Read the model definition and answer for the solid it produces. Units are mm, in the model's axes. A direction names the side the tool comes from. Give positions to 0.01 mm unless a question says otherwise; leave off trailing zeros. Loops run counter-clockwise (first coordinate to the right, second up) from the corner with the lowest first, then second, coordinate; pieces in that order, holes last. Notation, with made-up numbers: (36, 6.25) -> (79, 6.25) arc R23 cw to (79, 14.25) -> close; hole circle Ø9 at (42.25, 68.5). An arc over 180 degrees is marked (long way). Answer as CSV lines item,"result". Start each with the question number.
Autodesk Inventor part; units mm, degrees
ref_plane "YZ Plane" through (0, 0, 0) normal (1, 0, 0) x (0, 1, 0)
ref_plane "XZ Plane" through (0, 0, 0) normal (0, 1, 0) x (-1, 0, 0)
ref_plane "XY Plane" through (0, 0, 0) normal (0, 0, 1) x (1, 0, 0)
sketch "Sketch1" plane through (0, 0, 0) normal (0, 1, 0) x (-1, 0, 0)
  line L0 (0, 0) -> (60, 0)
  line L1 (60, 0) -> (60, -100)
  line L2 (60, -100) -> (0, -100)
  line L3 (0, -100) -> (0, 0)
  dimension "d0" = 100
  dimension "d1" = 60
extrude "Extrusion1" add sketch "Sketch1" along normal blind 40
sketch "Sketch2" plane through (0, 0, 0) normal (1, 0, 0) x (0, 0, -1)
  line L0 (0, 0) -> (37.6485, 44.8677)
  line L1 (0, 0) -> (58.5706, 0) construction
  line L2 (100, 40) -> (0, 40)
  line L3 (0, 40) -> (0, 0)
  point P0 (33.564, 40)
  dimension "d4" = 50
extrude "Extrusion2" cut sketch "Sketch2" against normal blind 70
sketch "Sketch3" plane through (0, 0, -100) normal (1, 0, 0) x (0, 0, -1)
  line L0 (0, 0) -> (-17, 0)
  line L1 (-100, 0) -> (0, 0)
  line L2 (0, 40) -> (-66.436, 40)
  line L3 (-17, 40) -> (-37, 40)
  line L4 (-37, 40) -> (-37, 10)
  line L5 (-37, 10) -> (-17, 10)
  line L6 (-17, 10) -> (-17, 40)
  dimension "d7" = 17
  dimension "d8" = 20
  dimension "d9" = 30
extrude "Extrusion3" add sketch "Sketch3" along normal blind 20
sketch "Sketch4" plane through (0, 10, -63) normal (0, 0, 1) x (1, 0, 0)
  line L0 (0, 30) -> (-60, 30)
  line L1 (0, 30) -> (29.4147, 5.3181)
  line L2 (0, 30) -> (38.3982, 30) construction
  line L3 (0, 30) -> (20, 30)
  line L4 (0, 30) -> (20, 30)
  line L5 (20, 30) -> (20, 13.218)
  line L6 (20, 0) -> (20, 30)
  point P0 (0, -10)
  dimension "d12" = 40
extrude "Extrusion4" cut sketch "Sketch4" against normal blind 61.75
ref_plane "Work Plane1" through (-30, 0, -100) normal (1, 0, 0) x (0, 0, -1)
mirror "Mirror1" about plane through (-30, 0, -100) normal (1, 0, 0) of "Extrusion3", "Extrusion4"
sketch "Sketch5" plane through (0, 40, -63) normal (0.6428, 0.766, 0) x (0.766, -0.6428, 0)
  circle A0 centre (12.5, 10) radius 5
  point P0 (25.7115, -63)
  dimension "d16" = 10
extrude "Extrusion5" cut sketch "Sketch5" against normal blind 27
mirror "Mirror2" about plane through (-30, 0, -100) normal (1, 0, 0) of "Extrusion5"
sketch "Sketch6" plane through (20, 10, -83) normal (0, 0, -1) x (-1, 0, 0)
  line L0 (20, 30) -> (20, 0)
  line L1 (20, 30) -> (20, 20)
  line L2 (20, 20) -> (18.6004, 20)
  line L3 (18.6004, 20) -> (18.6004, 28.8256)
  line L4 (0, 13.218) -> (20, 30)
  point P0 (20, -10)
  point P1 (20, 20)
  dimension "d19" = 10
extrude "Extrusion6" cut sketch "Sketch6" against normal blind 38.25
mirror "Mirror3" about plane through (-30, 0, -100) normal (1, 0, 0) of "Extrusion6"
properties part number "taslak"
(1) Find section B-B on y = 32. Give the number of separate pieces and of enclosed holes in the cut face, then the cut area to 3 significant figures.
(2) Find section A-A on x = -22.5. Write down the section's boundary in (y, z).
(3) Find section C-C on z = -48. Write down the section's boundary in (x, y).
(4) The mould has two halves that part along X. Classify faces 4 (the face through (-70, 21, -83)), 5 (the face through (-72.897, 29.178, -68.416)), 6 (the face through (1.4, 34, -73)): pulls with the +X half, pulls with the -X half, needs draft (parallel to the pull), parting line crosses it, or undercut.
(5) A tool of negligible diameter and unlimited length cuts with its end or side. For faces 1 (the face through (10, 10, -73)), 2 (the face through (-61.4, 34, -73)), 3 (the face through (10, 21, -83)), from which of +Z, -Z, +X, -X, +Y, -Y can it reach the whole face along a straight path? Write none if from no direction.
(6) Find the intervals of material crossed by line 1 along X through (y, z) = (13, -83.5); line 2 along Y through (x, z) = (6, -70); line 3 along Y through (x, z) = (1, -70), in increasing order. Write a range as from..to.
(7) Each of these flat-tipped pins is pushed along its axis until it touches: P1, Ø10, axis at x = -69, z = -72, coming from the -Y side; P2, Ø2.5, axis at y = 35, z = -69, coming from the -X side; P3, Ø0.7, axis at x = 0.5, z = -70.5, coming from the +Y side; P4, Ø20, axis at y = 11.5, z = -54.5, coming from the -X side. Where does it stop, or does it pass through?
Answer block:
1,separate pieces,"3"
1,enclosed holes,"0"
1,area,"4,610 mm2"
2,outline,"(0, -100) -> (40, -100) -> (40, -33.56) -> (0, 0) -> close"
3,outline,"(-60, 0) -> (0, 0) -> (0, 40) -> (-60, 40) -> close"
4,face 4,"needs draft"
4,face 5,"pulls with the -X half"
4,face 6,"undercut"
5,face 1,"+Z, -Z, +X, -Y"
5,face 2,"+Z, -Z, +Y"
5,face 3,"-Z, +X, +Y, -Y"
6,line 1,"x = -60..0"
6,line 2,"y = 10..21.48, 33.93..34.97"
6,line 3,"y = 10..15.52, 27.97..30"
7,P1,"stops at y = 10"
7,P2,"stops at x = -67.44"
7,P3,"stops at y = 30"
7,P4,"stops at x = -80"
